Part model, mm, in its own coordinate system. Give positions to 0.01 mm unless a question says otherwise; leave off trailing zeros. Loops run counter-clockwise (first coordinate to the right, second up) from the corner with the lowest first, then second, coordinate; pieces in that order, holes last. Notation, with made-up numbers: (64.25, 44) -> (100.25, 44) arc R24 cw to (100.25, 72) -> close; hole circle Ø8 at (-10, 6). An arc over 180 degrees is marked (long way). One line per question, with ' | ' between items.
```python
from build123d import *

# Parameters (mm, degrees)
SKETCH1_R                = 28.575
SKETCH1_R_2              = 25.4
BOSS_EXTRUDE1_DEPTH      = 15.24
BOSS_EXTRUDE2_START      = -15.24
BOSS_EXTRUDE2_DEPTH      = 15.24
FILLET1_R                = 25.4
CIRPATTERN1_COUNT        = 6
FILLET1_OF_CIRPATTERN1_R = 25.4
SKETCH3_R                = 2.2225
CUT_EXTRUDE1_DEPTH       = 49.331929565
CIRPATTERN2_COUNT        = 6


with BuildPart() as part:
    # Sketch1 → Boss-Extrude1 (new body)
    with BuildSketch(Plane(origin=(0, 0, 0), x_dir=(1, 0, 0), z_dir=(0, 1, 0))):
        with Locations(Location((0, 0, 0), (0, 0, 270))):
            Circle(SKETCH1_R)
        with Locations(Location((0, 0, 0), (0, 0, 270))):
            Circle(SKETCH1_R_2, mode=Mode.SUBTRACT)
    extrude(amount=BOSS_EXTRUDE1_DEPTH)

    # Sketch2 → Boss-Extrude2 (add)
    with BuildSketch(Plane(origin=(0, 15.24, 0), x_dir=(1, 0, 0), z_dir=(0, 1, 0)).offset(BOSS_EXTRUDE2_START)):
        with BuildLine():
            ThreePointArc((-28.0035, 5.686353203), (-34.29, 0), (-28.0035, -5.686353203))
            ThreePointArc((-28.0035, -5.686353203), (-28.575, 0), (-28.0035, 5.686353203))
        make_face()
    boss_extrude2 = extrude(amount=BOSS_EXTRUDE2_DEPTH)

    # Fillet1
    fillet1_edges = [part.edges().sort_by_distance(p)[0] for p in [
        (-28.0035, 7.62, -5.686353203),
        (-28.0035, 7.62, 5.686353203),
    ]]
    fillet(fillet1_edges, radius=FILLET1_R)

    # CirPattern1: Boss-Extrude2 ×6 about axis
    cirpattern1_axis = Axis((0, 0, 0), (0, 1, 0))
    for i in range(1, CIRPATTERN1_COUNT):
        add(boss_extrude2.rotate(cirpattern1_axis, i * 360 / CIRPATTERN1_COUNT))

    # Fillet1 of CirPattern1
    fillet1_of_cirpattern1_edges = [part.edges().sort_by_distance(p)[0] for p in [
        (-18.926276329, 7.62, 21.408565793),
        (-9.077223671, 7.62, 27.094918996),
        (9.077223671, 7.62, 27.094918996),
        (18.926276329, 7.62, 21.408565793),
        (28.0035, 7.62, 5.686353203),
        (28.0035, 7.62, -5.686353203),
        (18.926276329, 7.62, -21.408565793),
        (9.077223671, 7.62, -27.094918996),
        (-9.077223671, 7.62, -27.094918996),
        (-18.926276329, 7.62, -21.408565793),
    ]]
    fillet(fillet1_of_cirpattern1_edges, radius=FILLET1_OF_CIRPATTERN1_R)

    # Sketch3 → Cut-Extrude1 (cut, symmetric)
    with BuildSketch(Plane(origin=(0, 15.24, 0), x_dir=(1, 0, 0), z_dir=(0, 1, 0))):
        with Locations(Location((-29.845, 0, 0), (0, 0, 270))):
            Circle(SKETCH3_R)
    cut_extrude1 = extrude(amount=CUT_EXTRUDE1_DEPTH, both=True, mode=Mode.SUBTRACT)

    # CirPattern2: Cut-Extrude1 ×6 about axis
    cirpattern2_axis = Axis((0, 0, 0), (0, 1, 0))
    for i in range(1, CIRPATTERN2_COUNT):
        add(cut_extrude1.rotate(cirpattern2_axis, i * 360 / CIRPATTERN2_COUNT), mode=Mode.SUBTRACT)


solid = part.part
```
1) Saw through at C-C (y = 3.5). State how many separate pieces and enclosed holes the cut face has, and give its area (3 significant figures).
Found:
separate pieces: 1 | enclosed holes: 7 | area: 847 mm2
2) Pin check, flat tips, straight feed: P1, Ø4, axis at x = 3, y = 11.5, coming from the -Z side; P2, Ø8, axis at x = 26, y = 2, coming from the -Z side; P3, Ø1.5, axis at y = 12, z = -23.5, coming from the -X side. Stop position of each tip, or through.
Found:
P1: z = -28.56 | P2: z = -19.02 | P3: x = -20.59
3) Saw through at A-A (x = 0). Give the cut face in (y, z) (3 decimals), and give its area (3 significant figures).
Found:
outline: (0, -28.575) -> (15.24, -28.575) -> (15.24, -25.4) -> (0, -25.4) -> close; (0, 25.4) -> (15.24, 25.4) -> (15.24, 28.575) -> (0, 28.575) -> close | area: 96.8 mm2
4) Saw through at B-B (z = 0). Give the cut face in (x, y), and give its area (3 significant figures).
Found:
outline: (-34.29, 0) -> (-32.07, 0) -> (-32.07, 15.24) -> (-34.29, 15.24) -> close; (-27.62, 0) -> (-25.4, 0) -> (-25.4, 15.24) -> (-27.62, 15.24) -> close; (25.4, 0) -> (27.62, 0) -> (27.62, 15.24) -> (25.4, 15.24) -> close; (32.07, 0) -> (34.29, 0) -> (34.29, 15.24) -> (32.07, 15.24) -> close | area: 135 mm2
5) Drill centre lines: line 1 (X direction, y = 11, z = 0); line 2 (X direction, y = 7, z = -1); line 3 (Z direction, x = 15, y = 9.25). Where is each one in solid material? Low to high.
Found:
line 1: -34.29 to -32.07, -27.62 to -25.4, 25.4 to 27.62, 32.07 to 34.29 | line 2: -34.2 to -31.83, -27.86 to -25.38, 25.38 to 27.86, 31.83 to 34.2 | line 3: -30.42 to -28.07, -23.63 to -20.5, 20.5 to 23.63, 28.07 to 30.42
6) Pull direction Z, two halves, no side cores. Call faces 1 (the cylindrical face through (-0.025, 7.513, 28.575)), 2 (the cylindrical face through (24.759, 7.513, -14.266)), 3 (the cylindrical face through (12.95, 7.73, -24.82)), 4 (the flat face through (17.94, 0, -18.194)): pulls with the +Z half, pulls with the -Z half, needs draft (parallel to the pull), parting line crosses it, or undercut.
Found:
face 1: pulls with the +Z half | face 2: pulls with the -Z half | face 3: undercut | face 4: needs draft
